Model file for the job. Use its own axes, mm. Face numbers are marked on the shaded views. A direction names the side the tool comes from. Give positions to 0.01 mm unless a question says otherwise; leave off trailing zeros. Order: outer loops, then holes, each group sorted by start corner. A loop starts at its lowest first (then second) coordinate and runs counter-clockwise, first axis right, second up. Notation, with made-up numbers: (50, 30.25) -> (68, 30.25) arc R31 ccw to (68, 61.25) -> close; hole circle Ø6 at (29, 47). An arc over 180 degrees is marked (long way). Use CSV: the item, a comma, the result in double quotes. Start each with the question number.
1. Cut at B-B on x = 7. List the corners of the cut face in (y, z), then the cut area to 3 significant figures.
2. Cut at A-A on z = -9.25. List the corners of the cut face in (x, y), then the cut area to 3 significant figures.
3. Pull direction Z, two halves, no side cores. Call the marked faces 1, 2 and 3: released by +Z, released by -Z, zero draft, split by the parting line, or undercut.
4. Cut at C-C on y = 1.7. List the corners of the cut face in (x, z), then the cut area to 3 significant figures.
5. Drop a flat-ended pin along its axis: pin 1 (1.5 mm diameter, centred on x = 15, y = 1.5, fed in from -Z). Give the stop position or say it passes through.
6. Wall check: line 1 (X direction, y = 1, z = -17.75); line 2 (Z direction, x = 25, y = 2.95); line 3 (X direction, y = 1.65, z = -13.5). Give the ranges that are in metal, low to high. Write a range as from..to.
7. 3-axis set-ups, long thin cutter, end or side, ignore diameter. For the marked faces 4, 5 and 6: which of +Z, -Z, +X, -X, +Y, -Y reach the whole face in a straight line?
8. Cut at D-D on x = 21. List the corners of the cut face in (y, z), then the cut area to 3 significant figures.
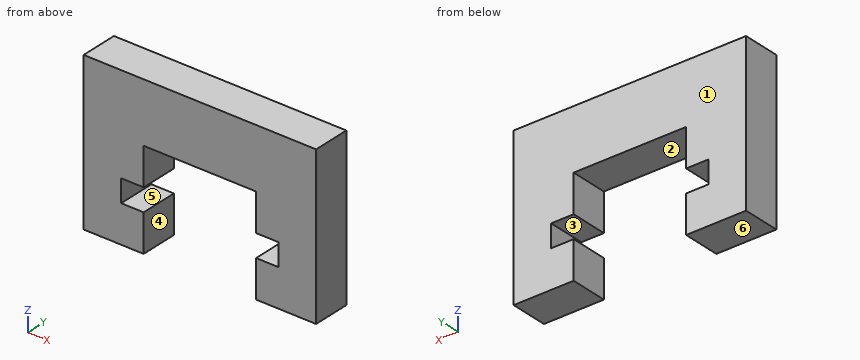
```python
from build123d import *

# Parameters (mm, degrees)
EXTRUDE_1_DEPTH     = 5
CUT_EXTRUDE_START   = -5
SKETCH_2_W          = 21
SKETCH_2_H          = 3
CUT_EXTRUDE_1_DEPTH = 5


with BuildPart() as part:
    # 草图1 → 凸台-拉伸1 (new body)
    with BuildSketch(Plane(origin=(0, 0, 0), x_dir=(1, 0, 0), z_dir=(0, 1, 0))):
        Polygon((0, 21), (0, 0), (31, 0), (31, 21), (23, 21), (23, 8), (8, 8), (8, 21), align=None)
    extrude(amount=EXTRUDE_1_DEPTH)

    # 草图2 → 切除-拉伸1 (cut)
    with BuildSketch(Plane(origin=(0, 5, 0), x_dir=(1, 0, 0), z_dir=(0, 1, 0)).offset(CUT_EXTRUDE_START)):
        with Locations((15.5, 14.5)):
            Rectangle(SKETCH_2_W, SKETCH_2_H)
    extrude(amount=CUT_EXTRUDE_1_DEPTH, mode=Mode.SUBTRACT)


solid = part.part
```
Verdict:
1,outline,"(0, -21) -> (5, -21) -> (5, -16) -> (0, -16) -> close; (0, -13) -> (5, -13) -> (5, 0) -> (0, 0) -> close"
1,area,"90.0 mm^2"
2,outline,"(0, 0) -> (8, 0) -> (8, 5) -> (0, 5) -> close; (23, 0) -> (31, 0) -> (31, 5) -> (23, 5) -> close"
2,area,"80.0 mm^2"
3,face 1,"zero draft"
3,face 2,"released by -Z"
3,face 3,"undercut"
4,outline,"(0, -21) -> (8, -21) -> (8, -16) -> (5, -16) -> (5, -13) -> (8, -13) -> (8, -8) -> (23, -8) -> (23, -13) -> (26, -13) -> (26, -16) -> (23, -16) -> (23, -21) -> (31, -21) -> (31, 0) -> (0, 0) -> close"
4,area,"438 mm^2"
5,pin 1,"z = -8"
6,line 1,"0..8, 23..31"
6,line 2,"-21..-16, -13..0"
6,line 3,"0..5, 26..31"
7,face 4,"-Z, +Y, -Y"
7,face 5,"+Y, -Y"
7,face 6,"-Z, +X, -X, +Y, -Y"
8,outline,"(0, -8) -> (5, -8) -> (5, 0) -> (0, 0) -> close"
8,area,"40.0 mm^2"
